Design review of the part built by this model. Coordinates are the model's own, in mm. A direction names the side the tool comes from. Coordinates: 2 decimals unless noted, no trailing zeros. Write each loop counter-clockwise with the first axis right and the second up, starting at its lowest first coordinate (ties: lowest second). Pieces come first, ordered by that corner, then holes. Notation, with made-up numbers: (-37, 7.5) - (21, 7.5) arc R33 ccw to (21, 38.5) - close; hole circle Ø6 at (-6.5, -28.75). An arc over 180 degrees is marked (long way). Use a Markdown table: item, result.
from build123d import *

# Parameters (mm, degrees)
F_01_BASE_PROFILE_W           = 110
F_01_BASE_PROFILE_H           = 34
F_01_BASE_PROFILE_R           = 3.5
F_01_BASE_EXTRUDE_DEPTH       = 18
F_02_BOSS_PROFILE_W           = 70
F_02_BOSS_PROFILE_H           = 20
F_02_REINFORCEMENT_BOSS_DEPTH = 26


with BuildPart() as part:
    # 01_Base_Profile → 01_Base_Extrude (new body)
    with BuildSketch(Plane(origin=(0, 0, 0), x_dir=(1, 0, 0), z_dir=(0, 1, 0))):
        Rectangle(F_01_BASE_PROFILE_W, F_01_BASE_PROFILE_H)
        with Locations(Location((-40, 0, 0), (0, 0, 270))):
            Circle(F_01_BASE_PROFILE_R, mode=Mode.SUBTRACT)
        with Locations(Location((40, 0, 0), (0, 0, 270))):
            Circle(F_01_BASE_PROFILE_R, mode=Mode.SUBTRACT)
    extrude(amount=F_01_BASE_EXTRUDE_DEPTH)

    # 02_Boss_Profile → 02_Reinforcement_Boss (add)
    with BuildSketch(Plane(origin=(0, 0, 0), x_dir=(1, 0, 0), z_dir=(0, 1, 0))):
        Rectangle(F_02_BOSS_PROFILE_W, F_02_BOSS_PROFILE_H)
    extrude(amount=F_02_REINFORCEMENT_BOSS_DEPTH)


solid = part.part
(1) Machinability: for faces 1 (the flat face through (35, 22, 0)), 2 (the flat face through (-35, 22, 0)), 3 (the flat face through (-55, 9, 0)), 4 (the flat face through (0, 22, 10)), 5 (the flat face through (0, 22, -10)), which of the approach directions +Z, -Z, +X, -X, +Y, -Y give a long, thin tool a straight path to every point of the face, cutting with its end or side? Answer none if there is none.
Determined:
| item | result |
|---|---|
| face 1 | +Z, -Z, +X, +Y |
| face 2 | +Z, -Z, -X, +Y |
| face 3 | +Z, -Z, -X, +Y, -Y |
| face 4 | +Z, +X, -X, +Y |
| face 5 | -Z, +X, -X, +Y |
(2) Take a section at A-A on x = 40. Write out the cut boundary in (y, z), and give its area (3 significant figures).
Determined:
| item | result |
|---|---|
| outline | (0, -17) - (18, -17) - (18, -3.5) - (0, -3.5) - close; (0, 3.5) - (18, 3.5) - (18, 17) - (0, 17) - close |
| area | 486 mm2 |
(3) For L1, parallel to X at y = 4.25, z = 0; L2, parallel to Z at x = 37, y = 16; L3, parallel to Y at x = -36.5, z = 11, list the stretches that pass through material, from the lowest coordinate up. Write a range as from..to.
Determined:
| item | result |
|---|---|
| L1 | -55..-43.5, -36.5..36.5, 43.5..55 |
| L2 | -17..-1.8, 1.8..17 |
| L3 | 0..18 |
(4) Take a section at C-C on z = 0. Write out the cut boundary in (x, y).
Determined:
| item | result |
|---|---|
| outline | (-55, 0) - (-43.5, 0) - (-43.5, 18) - (-55, 18) - close; (-36.5, 0) - (36.5, 0) - (36.5, 18) - (35, 18) - (35, 26) - (-35, 26) - (-35, 18) - (-36.5, 18) - close; (43.5, 0) - (55, 0) - (55, 18) - (43.5, 18) - close |
(5) Take a section at B-B on y = 3.5. Write out the cut boundary in (x, z).
Determined:
| item | result |
|---|---|
| outline | (-55, -17) - (55, -17) - (55, 17) - (-55, 17) - close; hole circle Ø7 at (-40, 0); hole circle Ø7 at (40, 0) |
(6) Take a section at D-D on z = 7. Write out the cut boundary in (x, y).
Determined:
| item | result |
|---|---|
| outline | (-55, 0) - (55, 0) - (55, 18) - (35, 18) - (35, 26) - (-35, 26) - (-35, 18) - (-55, 18) - close |
(7) Draft analysis for pull direction Z (two halves, no side actions). For faces 6 (the cylindrical face through (-36.53, 8.87, -0.46)), 7 (the flat face through (55, 9, 0)), 8 (the flat face through (-1, 9, -17)), state which applies: +Z half, -Z half, draft (parallel to the pull), parting line (faces both ways), or undercut.
Determined:
| item | result |
|---|---|
| face 6 | undercut |
| face 7 | draft |
| face 8 | -Z half |
(8) For pin 1 (1.5 mm diameter, centred on x = 31.5, y = 18.5, fed in from -Z); pin 2 (4 mm diameter, centred on x = -4, y = 24, fed in from -Z); pin 3 (2 mm diameter, centred on x = -38.5, z = -1, fed in from -Y); pin 4 (9 mm diameter, centred on x = -5.5, y = 23.5, fed in from +Z), all flat-tipped, find the tip position at first contact; note any pin that passes through.
Determined:
| item | result |
|---|---|
| pin 1 | z = -17 |
| pin 2 | z = -10 |
| pin 3 | through |
| pin 4 | z = 10 |
